```python
from build123d import *

# Parameters (mm, degrees)
SKETCH2_W           = 30
SKETCH2_H           = 44
BOSS_EXTRUDE1_DEPTH = 6
SKETCH4_W           = 10.879446424
SKETCH4_H           = 6.5
SKETCH4_W_2         = 8.120553576
SKETCH4_W_3         = 2.867356219
SKETCH4_W_4         = 16.132643781
BOSS_EXTRUDE2_DEPTH = 4.03177
SKETCH3_W           = 3.5
SKETCH3_H           = 44
SKETCH3_W_2         = 7
SKETCH3_H_2         = 6.8
CUT_EXTRUDE3_DEPTH  = 1
FILLET1_R           = 0.5
CUT_EXTRUDE4_REACH  = 8
SKETCH5_R           = 1.5
SKETCH6_R           = 1.5
CUT_EXTRUDE5_DEPTH  = 6


with BuildPart() as part:
    # Sketch2 → Boss-Extrude1 (new body)
    with BuildSketch(Plane(origin=(0, 1.96823021, 0), x_dir=(-1, 0, 0), z_dir=(0, -1, 0))):
        with Locations((-15, 0)):
            Rectangle(SKETCH2_W, SKETCH2_H)
    extrude(amount=BOSS_EXTRUDE1_DEPTH)

    # Sketch4 → Boss-Extrude2 (add)
    with BuildSketch(Plane(origin=(0, -4.03176979, 0), x_dir=(-1, 0, 0), z_dir=(0, -1, 0))):
        with Locations((-5.439723212, 25.25)):
            Rectangle(SKETCH4_W, SKETCH4_H)
        with Locations((-25.939723212, 25.25)):
            Rectangle(SKETCH4_W_2, SKETCH4_H)
        with Locations((-1.43367811, -25.25)):
            Rectangle(SKETCH4_W_3, SKETCH4_H)
        with Locations((-21.93367811, -25.25)):
            Rectangle(SKETCH4_W_4, SKETCH4_H)
    extrude(amount=-BOSS_EXTRUDE2_DEPTH)

    # Sketch3 → Cut-Extrude3 (cut)
    with BuildSketch(Plane(origin=(0, 1.96823021, 0), x_dir=(-1, 0, 0), z_dir=(0, -1, 0))):
        with Locations((-19.354808617, 0)):
            Rectangle(SKETCH3_W, SKETCH3_H)
        with Locations((-5.604808617, 3.1)):
            Rectangle(SKETCH3_W_2, SKETCH3_H_2)
        with Locations((-5.604808617, -11.9)):
            Rectangle(SKETCH3_W_2, SKETCH3_H_2)
        with Locations((-5.604808617, 18.1)):
            Rectangle(SKETCH3_W_2, SKETCH3_H_2)
    extrude(amount=CUT_EXTRUDE3_DEPTH, mode=Mode.SUBTRACT)

    # Fillet1
    fillet1_edges = [part.edges().sort_by_distance(p)[0] for p in [
        (0, -4.03176979, 0),
        (16.379446424, -4.03176979, -22),
        (5.439723212, -4.03176979, -28.5),
        (10.879446424, -4.03176979, -25.25),
        (10.879446424, -2.01588479, -28.5),
        (0, -2.01588479, -28.5),
        (21.879446424, -4.03176979, -25.25),
        (25.939723212, -4.03176979, -28.5),
        (21.879446424, -2.01588479, -28.5),
        (30, -2.01588479, -28.5),
        (2.867356219, -4.03176979, 25.25),
        (1.433678109, -4.03176979, 28.5),
        (2.867356219, -2.01588479, 22),
        (2.867356219, -2.01588479, 28.5),
        (0, -2.01588479, 28.5),
        (8.367356219, -4.03176979, 22),
        (21.933678109, -4.03176979, 28.5),
        (13.867356219, -4.03176979, 25.25),
        (13.867356219, -2.01588479, 28.5),
        (13.867356219, -2.01588479, 22),
        (30, -2.01588479, 28.5),
        (30, -4.03176979, 0),
        (0, 1.96823021, 0),
        (30, 1.96823021, 0),
    ]]
    fillet(fillet1_edges, radius=FILLET1_R)

    # Sketch5 → Cut-Extrude4 (cut, up to next)
    with BuildSketch(Plane(origin=(0, -4.03176979, 0), x_dir=(-1, 0, 0), z_dir=(0, -1, 0)), mode=Mode.PRIVATE) as cut_extrude4_sk1:
        with Locations((-5.439723212, 25.25)):
            Circle(SKETCH5_R)
    cut_extrude4_tool1 = extrude(cut_extrude4_sk1.sketch, amount=-CUT_EXTRUDE4_REACH, mode=Mode.PRIVATE) & part.part
    add(cut_extrude4_tool1.solids().sort_by_distance((5.439723, -4.03177, -25.25))[0], mode=Mode.SUBTRACT)
    # Sketch5 → Cut-Extrude4 (cut, up to next)
    with BuildSketch(Plane(origin=(0, -4.03176979, 0), x_dir=(-1, 0, 0), z_dir=(0, -1, 0)), mode=Mode.PRIVATE) as cut_extrude4_sk2:
        with Locations((-21.933678109, -25.25)):
            Circle(SKETCH5_R)
    cut_extrude4_tool2 = extrude(cut_extrude4_sk2.sketch, amount=-CUT_EXTRUDE4_REACH, mode=Mode.PRIVATE) & part.part
    add(cut_extrude4_tool2.solids().sort_by_distance((21.933678, -4.03177, 25.25))[0], mode=Mode.SUBTRACT)

    # Sketch6 → Cut-Extrude5 (cut)
    with BuildSketch(Plane.XZ.offset(4.03176979)):
        with Locations((14.104808617, -15)):
            Circle(SKETCH6_R)
        with Locations((14.104808617, 0)):
            Circle(SKETCH6_R)
        with Locations((14.104808617, 15)):
            Circle(SKETCH6_R)
    extrude(amount=-CUT_EXTRUDE5_DEPTH, mode=Mode.SUBTRACT)


solid = part.part
```
Can you work these out from the model? Positions are in its coordinate system, mm. A direction names the side the tool comes from. Round coordinates to 2 decimals unless told otherwise and drop trailing zeros. Loops run counter-clockwise (first coordinate to the right, second up) from the corner with the lowest first, then second, coordinate; pieces in that order, holes last. Notation, with made-up numbers: (8, 86.5) -> (35, 86.5) arc R26 cw to (35, 115.5) -> close; hole circle Ø9 at (4, -30.75). An arc over 180 degrees is marked (long way). One line per item, written item: value. Start each with the question number.
1. If we section it at B-B, the plane y = -2.05: Write out the boundary of the cut face in (x, z).
2. If I drill on probe 1 along X at (y, z) = (-0.95, -25.25); probe 2 along Z at (x, y) = (4.5, 1.5); probe 3 along Z at (x, y) = (15, -0.85), over which ranges is the centre line in solid material (lowest first)?
3. For faces 3 (the flat face through (26, 0, -25)), 4 (the flat face through (19, 0.968, 0)), 5 (the flat face through (6, 0.968, 12)), 6 (the flat face through (20, 0, 25)), 7 (the flat face through (10.879, -2, -25)), which set-ups out of +Z, -Z, +X, -X, +Y, -Y let a thin tool reach every point of the face, with its end or its side?
4. If we section it at C-C, the plane x = 7.5: Write out the boundary of the cut face in (y, z), then the cut area to 3 significant figures.
5. For pin 1 (1 mm diameter, centred on x = 1, z = 24, fed in from +Y); pin 2 (1.1 mm diameter, centred on x = 7, y = 1.5, fed in from -Z); pin 3 (1 mm diameter, centred on x = 19.5, z = 0, fed in from +Y), each with a flat end and sliding along its axis, tell me the tip position at first contact or that it passes through.
6. If we section it at A-A, the plane z = -25.25: Write out the boundary of the cut face in (x, y), then the cut area to 3 significant figures.
7. If we mould it in two halves opening along Z, with no side actions, what happens to faces 1 (the flat face through (5.7, 1.5, 0.3)), 2 (the flat face through (21.879, -2, -25))? For each: pulls with the +Z half, pulls with the -Z half, needs draft (parallel to the pull), parting line crosses it, or undercut.
8. If we section it at D-D, the plane z = 6: Write out the boundary of the cut face in (x, y).
Calculated:
1. outline: (0, -28) arc R0.5 ccw to (0.5, -28.5) -> (10.38, -28.5) arc R0.5 ccw to (10.88, -28) -> (10.88, -22) -> (21.88, -22) -> (21.88, -28) arc R0.5 ccw to (22.38, -28.5) -> (29.5, -28.5) arc R0.5 ccw to (30, -28) -> (30, 28) arc R0.5 ccw to (29.5, 28.5) -> (14.37, 28.5) arc R0.5 ccw to (13.87, 28) -> (13.87, 22.5) arc R0.5 cw to (13.37, 22) -> (3.37, 22) arc R0.5 cw to (2.87, 22.5) -> (2.87, 28) arc R0.5 ccw to (2.37, 28.5) -> (0.5, 28.5) arc R0.5 ccw to (0, 28) -> close; hole circle Ø3 at (5.44, -25.25); hole circle Ø3 at (14.1, -15); hole circle Ø3 at (14.1, 0); hole circle Ø3 at (14.1, 15); hole circle Ø3 at (21.93, 25.25)
2. probe 1: x = 0 to 3.94, 6.94 to 10.88, 21.88 to 30
2. probe 2: z = -22 to -21.5, -14.7 to -6.5, 0.3 to 8.5, 15.3 to 22
2. probe 3: z = -22 to -16.2, -13.8 to -1.2, 1.2 to 13.8, 16.2 to 28.5
3. face 3: -Z, +X, -X, +Y
3. face 4: +Z, -Z, +Y
3. face 5: +Y
3. face 6: +Z, +X, -X, +Y
3. face 7: -Z, +Y, -Y
4. outline: (-4.03, -28) arc R0.5 ccw to (-3.53, -28.5) -> (0, -28.5) -> (0, -22) -> (1.97, -22) -> (1.97, -21.5) -> (0.97, -21.5) -> (0.97, -14.7) -> (1.97, -14.7) -> (1.97, -6.5) -> (0.97, -6.5) -> (0.97, 0.3) -> (1.97, 0.3) -> (1.97, 8.5) -> (0.97, 8.5) -> (0.97, 15.3) -> (1.97, 15.3) -> (1.97, 22) -> (-3.53, 22) arc R0.5 ccw to (-4.03, 21.5) -> close
4. area: 270 mm²
5. pin 1: stops at y = 0
5. pin 2: stops at z = -22
5. pin 3: stops at y = 0.97
6. outline: (0, -3.53) arc R0.5 ccw to (0.5, -4.03) -> (3.94, -4.03) -> (3.94, 0) -> (0, 0) -> close; (6.94, -4.03) -> (10.38, -4.03) arc R0.5 ccw to (10.88, -3.53) -> (10.88, 0) -> (6.94, 0) -> close; (21.88, -3.53) arc R0.5 ccw to (22.38, -4.03) -> (29.5, -4.03) arc R0.5 ccw to (30, -3.53) -> (30, 0) -> (21.88, 0) -> close
6. area: 64.3 mm²
7. face 1: undercut
7. face 2: needs draft
8. outline: (0, -3.53) arc R0.5 ccw to (0.5, -4.03) -> (29.5, -4.03) arc R0.5 ccw to (30, -3.53) -> (30, 1.47) arc R0.5 ccw to (29.5, 1.97) -> (21.1, 1.97) -> (21.1, 0.97) -> (17.6, 0.97) -> (17.6, 1.97) -> (0.5, 1.97) arc R0.5 ccw to (0, 1.47) -> close
